For this review, take the finished solid that the model builds, in its own axes (mm). Round coordinates to 2 decimals unless told otherwise and drop trailing zeros. Write each loop counter-clockwise with the first axis right and the second up, starting at its lowest first coordinate (ties: lowest second). Pieces come first, ordered by that corner, then holes. Notation, with made-up numbers: (31.5, 6) -> (55.5, 6) arc R14 cw to (55.5, 16) -> close; hole circle Ø11 at (42.25, -27.75). An arc over 180 degrees is marked (long way). Answer in a Markdown table with one row per item.
from build123d import *

# Parameters (mm, degrees)
SKETCH015_R       = 0.5
PAD004_DEPTH      = 7.25
PAD004_DEPTH_BACK = 3.1
SKETCH016_R       = 0.5
PAD005_DEPTH      = 9.05
POCKET009_DEPTH   = 3.5


with BuildPart() as part:
    # Sketch015 → Pad004 (new body, two sides)
    with BuildSketch(Plane.XY) as pad004_sk:
        Circle(SKETCH015_R)
    extrude(amount=PAD004_DEPTH)
    extrude(pad004_sk.sketch, amount=-PAD004_DEPTH_BACK)

    # Sketch016 → Pad005 (join)
    with BuildSketch(Plane.XZ):
        with Locations((0, 7.25)):
            Circle(SKETCH016_R)
    extrude(amount=PAD005_DEPTH)

    # Sketch017 (on DatumPlane) → Pocket009 (cut)
    with BuildSketch(Plane.XZ.offset(9.05)):
        with BuildLine():
            ThreePointArc((-0.449305, 7.225), (0, 6.8), (0.449305, 7.225))
            Line((0.449305, 7.225), (0.499875, 7.225))
            ThreePointArc((0.499875, 7.225), (0.5005, 7.25), (0.499875, 7.275))
            Line((0.449305, 7.275), (0.499875, 7.275))
            ThreePointArc((0.449305, 7.275), (0, 7.7), (-0.449305, 7.275))
            Line((-0.499875, 7.275), (-0.449305, 7.275))
            ThreePointArc((-0.499875, 7.275), (-0.5005, 7.25), (-0.499875, 7.225))
            Line((-0.499875, 7.225), (-0.449305, 7.225))
        make_face()
    extrude(amount=-POCKET009_DEPTH, mode=Mode.SUBTRACT)


solid = part.part
1) Mouldability with a two-part tool opening along Z and no side actions: class faces 1 (the cylindrical face through (0.477, -4.462, 7.4)), 2 (the flat face through (0, 0, -3.1)), 3 (the cylindrical face through (-0.108, -0.488, 2.147)), 4 (the flat face through (0, -5.55, 7)) as pulls with the +Z half, pulls with the -Z half, needs draft (parallel to the pull), parting line crosses it, or undercut.
Solved:
| item | result |
|---|---|
| face 1 | parting line crosses it |
| face 2 | pulls with the -Z half |
| face 3 | needs draft |
| face 4 | undercut |
2) Clearance check with a flat-ended pin moving along its axis: pin 1 Ø4 at (y, z) = (-3.5, 3) entering from +X. State where the tip first meets the part, or that it passes through.
Solved:
| item | result |
|---|---|
| pin 1 | through |
3) Consider section C-C on z = 5.25. State the section outline as (x, y) points, then the cut area to 3 significant figures.
Solved:
| item | result |
|---|---|
| outline | circle Ø1 at (0, 0) |
| area | 0.785 mm² |
4) For line 1 (Z direction, x = -0.05, y = -2.75); line 2 (X direction, y = -0.25, z = 7); line 3 (Y direction, x = 0.2, z = -2.5), list the stretches that pass through material, from the lowest coordinate up. Write a range as [from, to].
Solved:
| item | result |
|---|---|
| line 1 | [6.75, 7.75] |
| line 2 | [-0.43, 0.43] |
| line 3 | [-0.46, 0.46] |
5) Consider section A-A on y = -6.25. State the section outline as (x, z) points (3 decimals).
Solved:
| item | result |
|---|---|
| outline | (-0.499, 7.225) arc R0.5 ccw to (0.499, 7.225) -> (0.449, 7.225) arc R0.45 cw to (-0.449, 7.225) -> close; (-0.499, 7.275) -> (-0.449, 7.275) arc R0.45 cw to (0.449, 7.275) -> (0.499, 7.275) arc R0.5 ccw to start |
6) Consider section B-B on x = 0. State the section outline as (y, z) points, then the cut area to 3 significant figures.
Solved:
| item | result |
|---|---|
| outline | (-9.05, 6.75) -> (-0.5, 6.75) -> (-0.5, -3.1) -> (0.5, -3.1) -> (0.5, 7.25) -> (0, 7.25) -> (0, 7.75) -> (-9.05, 7.75) -> (-9.05, 7.7) -> (-5.55, 7.7) -> (-5.55, 6.8) -> (-9.05, 6.8) -> close |
| area | 16.0 mm² |
7) Consider section D-D on y = -4. State the section outline as (x, z) points.
Solved:
| item | result |
|---|---|
| outline | circle Ø1 at (0, 7.25) |
